For this review, take the finished solid that the model builds, in its own axes (mm). A direction names the side the tool comes from. Round coordinates to 2 decimals unless told otherwise and drop trailing zeros. Order: outer loops, then holes, each group sorted by start corner. A loop starts at its lowest first (then second) coordinate and runs counter-clockwise, first axis right, second up. Notation, with made-up numbers: (62, -13) - (110, -13) arc R34 cw to (110, 19) - close; hole circle Ø11 at (-21, 54). An arc over 180 degrees is marked (long way). One line per item, written item: value.
```python
from build123d import *

# Parameters (mm, degrees)
EXTRUDE_1_OUTLINE_R      = 19
EXTRUDE_1_DEPTH          = 3
CUT_EXTRUDE_1_DEPTH      = 28.037011669
CUT_EXTRUDE_START        = -3
SKETCH_5_R               = 19
SKETCH_5_R_2             = 15
CUT_EXTRUDE_2_DEPTH      = 3
PATTERN_CIRCULAR_1_COUNT = 17
CUT_EXTRUDE_4_DEPTH      = 3
EXTRUDE_3_DEPTH          = 3
SKETCH_7_R               = 2
CUT_EXTRUDE_3_DEPTH      = 3


# Read off the part's stored shape, not the designer's step: 凸台-拉伸1
with BuildPart() as part:
    # 凸台-拉伸1 outline → 凸台-拉伸1 (new body)
    with BuildSketch(Plane.XY):
        Circle(EXTRUDE_1_OUTLINE_R)
    extrude(amount=EXTRUDE_1_DEPTH)

    # 草图2 → 切除-拉伸1 (cut, through all)
    with BuildSketch(Plane.XY):
        with BuildLine():
            ThreePointArc((1, 11.958260743), (0, 12), (-1, 11.958260743))
            add(Edge.make_bspline(
                [(-1, 11.958260743), (-0.697871553, 13.823728022), (-2.422759286, 14.803048248)],
                knots=[0, 0, 0, 1, 1, 1], degree=2))
            ThreePointArc((-2.422759286, 14.803048248), (0, 15), (2.422759286, 14.803048248))
            add(Edge.make_bspline(
                [(1, 11.958260743), (0.697871553, 13.823728022), (2.422759286, 14.803048248)],
                knots=[0, 0, 0, 1, 1, 1], degree=2))
        make_face()
    cut_extrude_1 = extrude(amount=CUT_EXTRUDE_1_DEPTH, mode=Mode.SUBTRACT)

    # 草图5 → 切除-拉伸2 (cut)
    with BuildSketch(Plane.XY.offset(3).offset(CUT_EXTRUDE_START)):
        Circle(SKETCH_5_R)
        Circle(SKETCH_5_R_2, mode=Mode.SUBTRACT)
    extrude(amount=CUT_EXTRUDE_2_DEPTH, mode=Mode.SUBTRACT)

    # 阵列(圆周)1: 切除-拉伸1 ×17 about axis
    pattern_circular_1_axis = Axis((0, 0, 3), (0, 0, -1))
    for i in range(1, PATTERN_CIRCULAR_1_COUNT):
        add(cut_extrude_1.rotate(pattern_circular_1_axis, i * 360 / PATTERN_CIRCULAR_1_COUNT), mode=Mode.SUBTRACT)

    # 草图8 → 切除-拉伸4 (cut)
    with BuildSketch(Plane(origin=(0, 0, 0), x_dir=(-1, 0, 0), z_dir=(0, 0, -1))):
        with BuildLine():
            Line((10.120821448, 11.071087264), (8.096657158, 8.856869812))
            ThreePointArc((8.096657158, 8.856869812), (6.278516295, -10.226447728), (-11.561990246, -3.212535065))
            Line((-11.561990246, -3.212535065), (-13.925196787, -5.575741606))
            ThreePointArc((-13.925196787, -5.575741606), (8.538005961, -12.332982373), (10.120821448, 11.071087264))
        make_face()
    extrude(amount=-CUT_EXTRUDE_4_DEPTH, mode=Mode.SUBTRACT)

    # 草图6 → 凸台-拉伸3 (add)
    with BuildSketch(Plane.XY.offset(3)):
        with BuildLine():
            Line((-30, 4), (0, 4))
            Line((0, 4), (0, -4))
            Line((0, -4), (-30, -4))
            ThreePointArc((-30, -4), (-34, 0), (-30, 4))
        make_face()
    extrude(amount=-EXTRUDE_3_DEPTH)

    # 草图7 → 切除-拉伸3 (cut)
    with BuildSketch(Plane(origin=(0, 0, 0), x_dir=(-1, 0, 0), z_dir=(0, 0, -1))):
        Circle(SKETCH_7_R)
        with Locations((30, 0)):
            Circle(SKETCH_7_R)
    extrude(amount=-CUT_EXTRUDE_3_DEPTH, mode=Mode.SUBTRACT)


solid = part.part
```
Item 1: Take a section at C-C (x = -23). Write out the cut boundary in (y, z).
Returned:
outline: (-4, 0) - (4, 0) - (4, 3) - (-4, 3) - close
Item 2: Machinability: for faces 4 (the cylindrical face through (-31.908, 0.601, 1.479)), 5 (the flat face through (-21, 4, 2)), 6 (the flat face through (-21, -4, 2)), which of the approach directions +Z, -Z, +X, -X, +Y, -Y give a long, thin tool a straight path to every point of the face, cutting with its end or side? Answer none if there is none.
Returned:
face 4: +Z, -Z
face 5: +Z, -Z, -X, +Y
face 6: +Z, -Z, -X, -Y
Item 3: For P1, Ø2.5, axis at x = -30, y = 0, coming from the -Z side; P2, Ø1.5, axis at y = -2.5, z = 0.5, coming from the +X side; P3, Ø0.9, axis at x = -21.5, z = 2, coming from the -Y side, all flat-tipped, find the tip position at first contact; note any pin that passes through.
Returned:
P1: through
P2: x = 14.87
P3: y = -4
Item 4: Take a section at B-B (y = -0.5). Count the separate pieces of the cut face and the enclosed holes in it, plus the area to 3 significant figures.
Returned:
separate pieces: 3
enclosed holes: 0
area: 122 mm^2
Item 5: Take a section at D-D (y = 5.75). Write out the cut boundary in (x, z).
Returned:
outline: (-10.53, 0) - (10.53, 0) - (10.53, 3) - (-10.53, 3) - close
Item 6: The part is to be moulded in two halves that separate along Y. For faces 1 (the cylindrical face through (-34, 0, 2)), 2 (the cylindrical face through (8.095, 8.859, 1.479)), 3 (the flat face through (-4, 2, 0)), say which applies: +Y half, -Y half, draft (parallel to the pull), parting line (faces both ways), or undercut.
Returned:
face 1: parting line
face 2: undercut
face 3: draft
Item 7: Take a section at A-A (x = 0). Write out the cut boundary in (y, z).
Returned:
outline: (-12, 0) - (-2, 0) - (-2, 3) - (-12, 3) - close; (2, 0) - (12, 0) - (12, 3) - (2, 3) - close
Item 8: Wall thickness on line 1 (Y direction, x = -30, z = 1.9); line 2 (X direction, y = -0.75, z = 0.5); line 3 (X direction, y = -1.75, z = 2.5): over which ranges is each line inside the solid? List them lowest first.
Returned:
line 1: -4 to -2, 2 to 4
line 2: -33.93 to -31.85, -28.15 to -1.85, 1.85 to 14.74
line 3: -33.6 to -30.97, -29.03 to -0.97, 0.97 to 14.87
